Can you work these out from the drawing? Everything is in mm from the part's minimum corner. A direction names the side the tool comes from. Round coordinates to 2 decimals unless told otherwise and drop trailing zeros. Order: outer loops, then holes, each group sorted by start corner. A loop starts at its lowest first (then second) coordinate and runs counter-clockwise, first axis right, second up. Notation, with made-up numbers: M 14,55.5 L 43,55.5 A17 ccw 43,87.5 Z; hole C -19,62.25 d2. An arc over 180 degrees is marked long. Write each question's results on one line, items separated by ' | '. Start each with the question number.
1. Suppose I cut it at D-D on z = 2. Write out the boundary of the cut face in (x, y) (1 decimal), and give its area (3 significant figures).
2. For the marked faces 1 and 2, which set-ups out of +Z, -Z, +X, -X, +Y, -Y let a thin tool reach every point of the face, with its end or its side?
3. We'd pull the mould along X, two halves only. Please class the marked faces 3, 4, 5 and 6: released by +X, released by -X, zero draft, split by the parting line, or undercut.
4. Suppose I cut it at B-B on y = 32. Write out the boundary of the cut face in (x, z) (1 decimal), and give its area (3 significant figures).
5. Please list where these lines run through material, in increasing order: L1, parallel to X at y = 18.5, z = 4.75; L2, parallel to X at y = 6, z = 9 (1 decimal); L3, parallel to Y at x = 47.5, z = 7.75.
6. Suppose I cut it at C-C on x = 44. Write out the boundary of the cut face in (y, z) (1 decimal).
7. I'm going to push flat-ended pins straight in: pin 1 (3 mm diameter, centred on x = 53, y = 6, fed in from +Z); pin 2 (3 mm diameter, centred on x = 11.875, y = 7.175, fed in from -Z). Where does each tip first touch, or does it pass through?
8. Suppose I cut it at A-A on z = 6. Write out the boundary of the cut face in (x, y) (1 decimal), and give its area (3 significant figures).
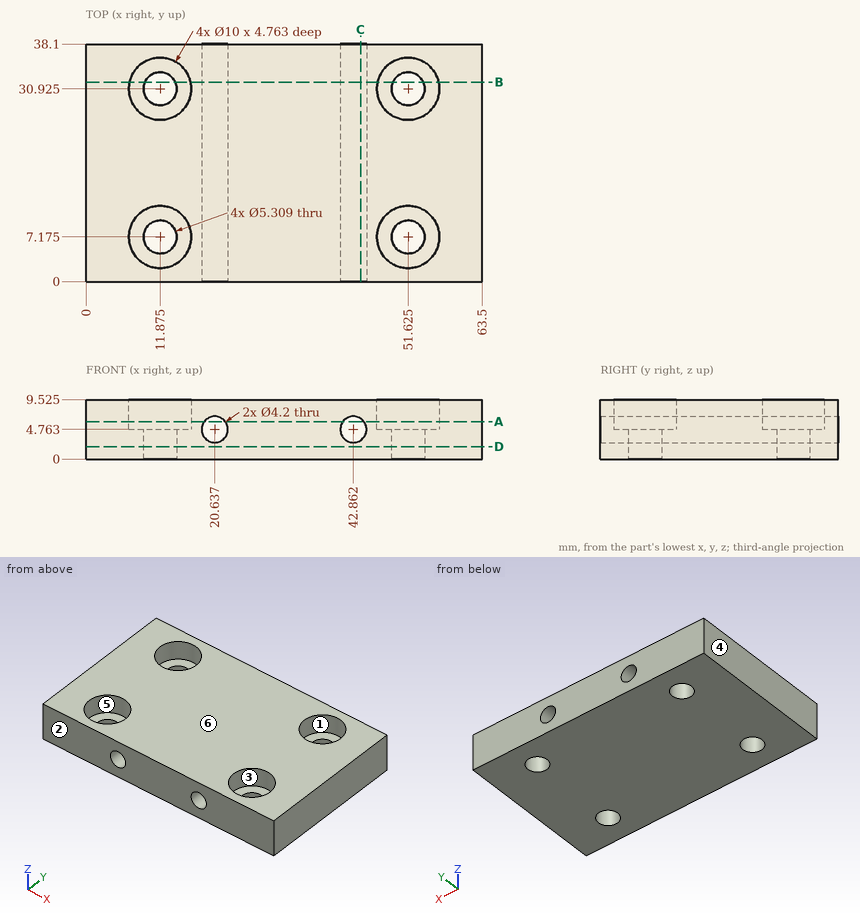
Filled sheet:
1) outline: M 0,0 L 63.5,0 L 63.5,38.1 L 0,38.1 Z; hole C 11.9,7.2 d5.3; hole C 11.9,30.9 d5.3; hole C 51.6,7.2 d5.3; hole C 51.6,30.9 d5.3 | area: 2,330 mm^2
2) face 1: +Z | face 2: +Z, -Z, +X, -X, -Y
3) face 3: undercut | face 4: released by -X | face 5: undercut | face 6: zero draft
4) outline: M 0,0 L 9.4,0 L 9.4,4.8 L 7,4.8 L 7,9.5 L 0,9.5 Z; M 14.3,0 L 49.2,0 L 49.2,4.8 L 46.7,4.8 L 46.7,9.5 L 16.8,9.5 L 16.8,4.8 L 14.3,4.8 Z; M 54.1,0 L 63.5,0 L 63.5,9.5 L 56.5,9.5 L 56.5,4.8 L 54.1,4.8 Z; hole C 20.6,4.8 d4.2; hole C 42.9,4.8 d4.2 | area: 438 mm^2
5) L1: x = 0 to 18.54, 22.74 to 40.76, 44.96 to 63.5 | L2: x = 0 to 7, 16.7 to 46.8, 56.5 to 63.5 | L3: y = 0 to 4.35, 10 to 28.1, 33.75 to 38.1
6) outline: M 0,0 L 38.1,0 L 38.1,3 L 0,3 Z; M 0,6.5 L 38.1,6.5 L 38.1,9.5 L 0,9.5 Z
7) pin 1: stops at z = 4.76 | pin 2: passes through
8) outline: M 0,0 L 18.9,0 L 18.9,38.1 L 0,38.1 Z; M 22.3,0 L 41.2,0 L 41.2,38.1 L 22.3,38.1 Z; M 44.6,0 L 63.5,0 L 63.5,38.1 L 44.6,38.1 Z; hole C 11.9,7.2 d10; hole C 11.9,30.9 d10; hole C 51.6,7.2 d10; hole C 51.6,30.9 d10 | area: 1,850 mm^2
